The figure shows three views and two pictorial views of one solid part (mm, origin at its lowest corner). Answer the questions. Round coordinates to 2 decimals unless told otherwise and drop trailing zeros. Order: outer loops, then holes, each group sorted by start corner. A loop starts at its lowest first (then second) coordinate and runs counter-clockwise, first axis right, second up. Notation, with made-up numbers: M 0,36 L 38,36 A18 cw 38,63 Z; hole C -15.5,-21.75 d9. An arc over 180 degrees is marked long. Answer as CSV lines item,"result".
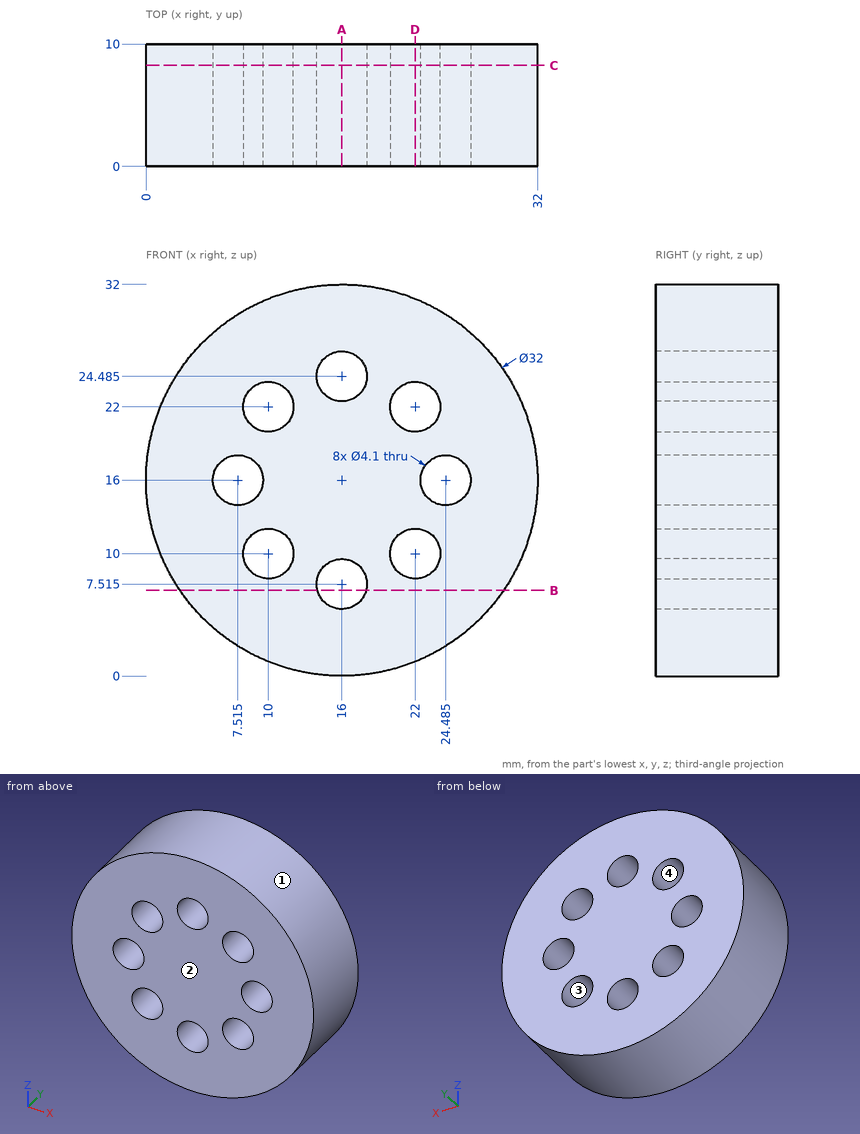
Item 1: Determine the mould class of the marked faces 1, 2, 3 and 4 for opening direction Z: +Z half, -Z half, draft (parallel to the pull), parting line (faces both ways), or undercut.
Ans:
face 1,"parting line"
face 2,"draft"
face 3,"undercut"
face 4,"undercut"
Item 2: A cutting plane is placed at D-D, the plane x = 22. Determine the outline of the cut face in (y, z).
Ans:
outline,"M 0,1.17 L 10,1.17 L 10,7.95 L 0,7.95 Z; M 0,12.05 L 10,12.05 L 10,19.95 L 0,19.95 Z; M 0,24.05 L 10,24.05 L 10,30.83 L 0,30.83 Z"
Item 3: A cutting plane is placed at C-C, the plane y = 8.25. Give the number of separate pieces and of enclosed holes in the cut face, and give its area (3 significant figures).
Ans:
separate pieces,"1"
enclosed holes,"8"
area,"699 mm2"
Item 4: A cutting plane is placed at B-B, the plane z = 7. Determine the outline of the cut face in (x, y), and give its area (3 significant figures).
Ans:
outline,"M 2.77,0 L 14.02,0 L 14.02,10 L 2.77,10 Z; M 17.98,0 L 29.23,0 L 29.23,10 L 17.98,10 Z"
area,"225 mm2"
Item 5: Find the intervals of material crossed by probe 1 along Z at (x, y) = (22, 7.25); probe 2 along Z at (x, y) = (11.5, 3) (1 decimal); probe 3 along X at (y, z) = (5.5, 15) (1 decimal), in increasing order. Write a range as [from, to].
Ans:
probe 1,"[1.17, 7.95], [12.05, 19.95], [24.05, 30.83]"
probe 2,"[0.6, 8.6], [11.4, 20.6], [23.4, 31.4]"
probe 3,"[0, 5.7], [9.3, 22.7], [26.3, 32]"
Item 6: A cutting plane is placed at A-A, the plane x = 16. Determine the outline of the cut face in (y, z) (1 decimal), and give its area (3 significant figures).
Ans:
outline,"M 0,0 L 10,0 L 10,5.5 L 0,5.5 Z; M 0,9.6 L 10,9.6 L 10,22.4 L 0,22.4 Z; M 0,26.5 L 10,26.5 L 10,32 L 0,32 Z"
area,"238 mm2"
Item 7: Flat-ended cylindrical pins translate along their axes: pin 1 (6 mm diameter, centred on y = 1.5, z = 4, fed in from -X); pin 2 (4 mm diameter, centred on x = 26.5, y = 3, fed in from -Z) (1 decimal); pin 3 (4.5 mm diameter, centred on x = 22, z = 22, fed in from +Y); pin 4 (3 mm diameter, centred on x = 20, y = 1.5, fed in from -Z). Find the tip coordinate at first contact, or state that the pin passes through.
Ans:
pin 1,"x = 2.77"
pin 2,"z = 2.4"
pin 3,"y = 10"
pin 4,"z = 0.2"
